Geometry: see drawing. Coordinates: mm, zero at the bounding-box minimum. Round coordinates to 2 decimals unless told otherwise and drop trailing zeros. Order: outer loops, then holes, each group sorted by start corner. A loop starts at its lowest first (then second) coordinate and runs counter-clockwise, first axis right, second up. Notation, with made-up numbers: (-11.75, 29.5) -> (-1.75, 29.5) arc R21 ccw to (-1.75, 46.5) -> close; hole circle Ø8 at (55.5, 42.5). An arc over 180 degrees is marked (long way). Write item = value, one per line. Start each with the question number.
(1) Ray query, line 1 (X direction, y = 3.1, z = 47); line 2 (Z direction, x = 20, y = 2.85); line 3 (Z direction, x = 19.25, y = 2.7). Return the intervals inside material, ascending.
(2) Draft query along X for the marked faces 1, 2 and 3. Return one class per face: released by +X, released by -X, zero draft, split by the parting line, or undercut.
(3) Cut plane C-C on y = 4. Return the cut outline in (x, z), then the cut area to 3 significant figures.
(4) Cut plane B-B on x = 20. Return the cut outline in (y, z), then the cut area to 3 significant figures.
(5) Cut plane A-A on z = 3. Return the cut outline in (x, y), then the cut area to 3 significant figures.
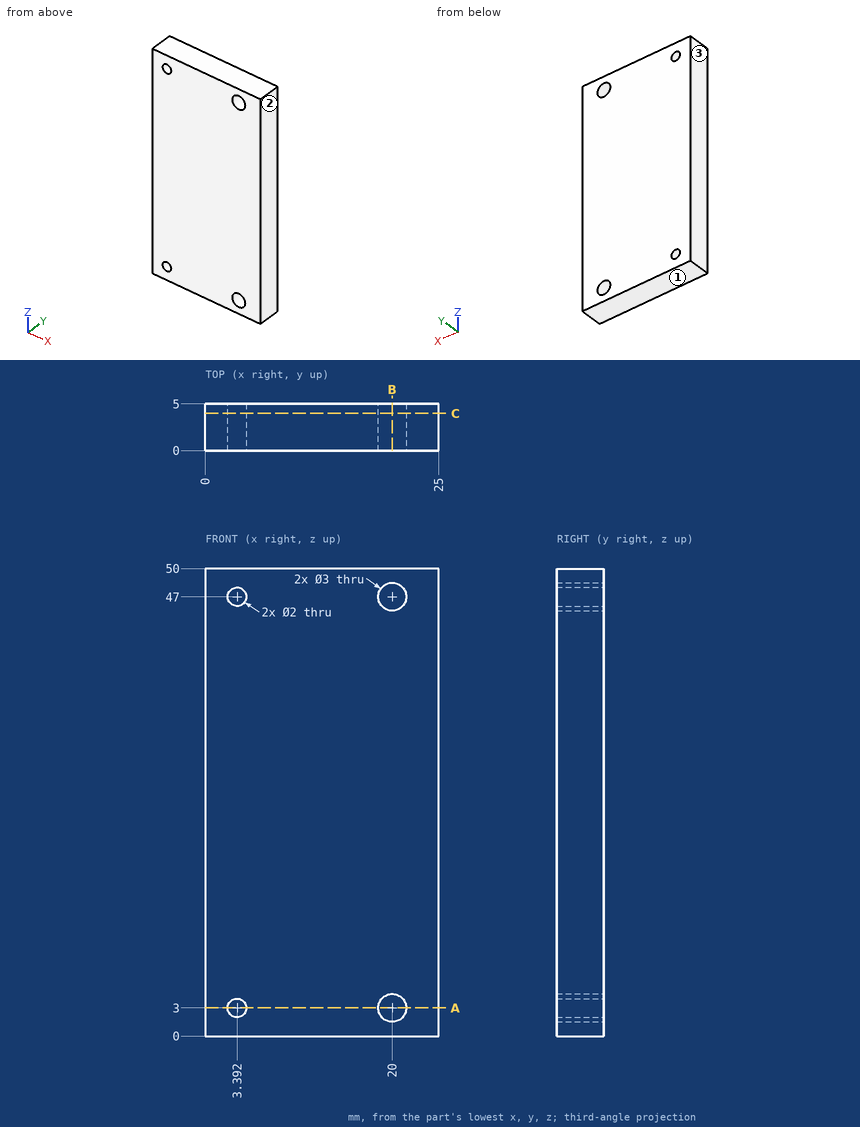
Evaluation:
q1.line_1 = 0 to 2.39, 4.39 to 18.5, 21.5 to 25
q1.line_2 = 0 to 1.5, 4.5 to 45.5, 48.5 to 50
q1.line_3 = 0 to 1.7, 4.3 to 45.7, 48.3 to 50
q2.face_1 = zero draft
q2.face_2 = released by +X
q2.face_3 = released by -X
q3.outline = (0, 0) -> (25, 0) -> (25, 50) -> (0, 50) -> close; hole circle Ø2 at (3.39, 3); hole circle Ø2 at (3.39, 47); hole circle Ø3 at (20, 3); hole circle Ø3 at (20, 47)
q3.area = 1,230 mm^2
q4.outline = (0, 0) -> (5, 0) -> (5, 1.5) -> (0, 1.5) -> close; (0, 4.5) -> (5, 4.5) -> (5, 45.5) -> (0, 45.5) -> close; (0, 48.5) -> (5, 48.5) -> (5, 50) -> (0, 50) -> close
q4.area = 220 mm^2
q5.outline = (0, 0) -> (2.39, 0) -> (2.39, 5) -> (0, 5) -> close; (4.39, 0) -> (18.5, 0) -> (18.5, 5) -> (4.39, 5) -> close; (21.5, 0) -> (25, 0) -> (25, 5) -> (21.5, 5) -> close
q5.area = 100 mm^2
